The figure shows three views and two pictorial views of one solid part (mm, origin at its lowest corner). Answer the questions. Coordinates: 2 decimals unless noted, no trailing zeros. Order: outer loops, then holes, each group sorted by start corner. A loop starts at its lowest first (then second) coordinate and runs counter-clockwise, first axis right, second up. Notation, with made-up numbers: (80, 76.5) -> (111, 76.5) arc R32 ccw to (111, 105.5) -> close; hole circle Ø2 at (62.5, 20). An arc over 180 degrees is marked (long way). Use one line per item in the form item = value.
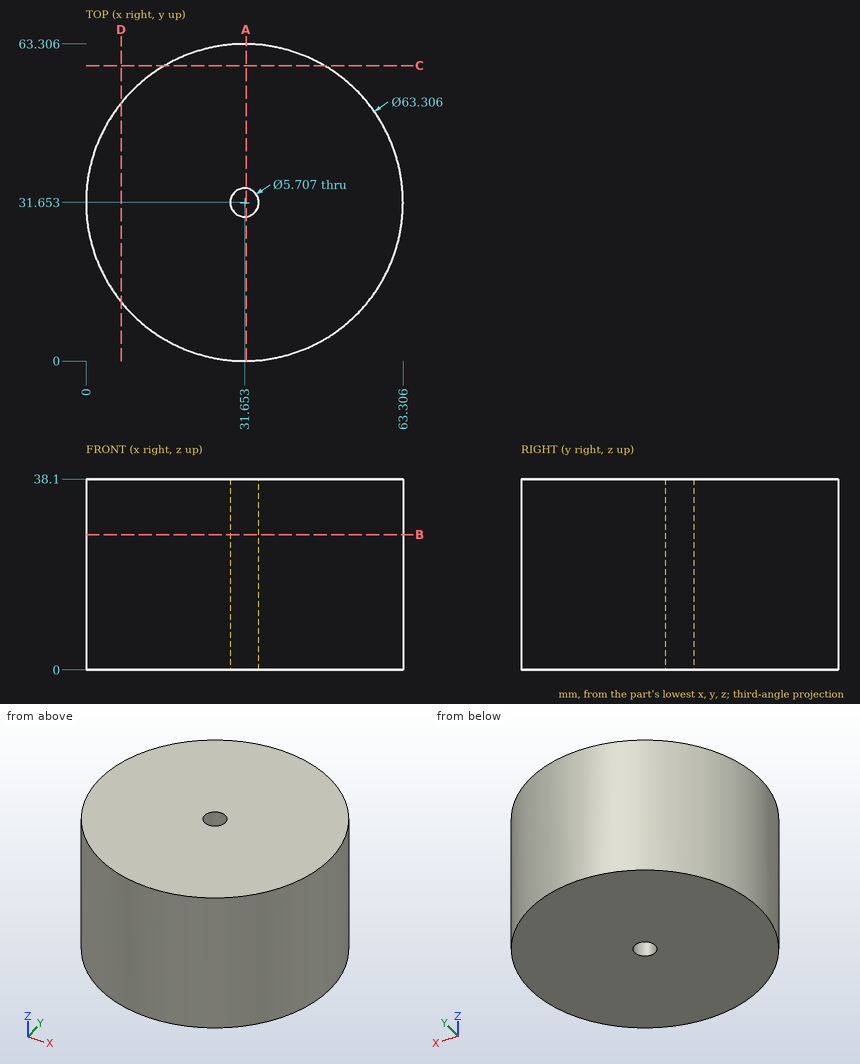
(1) Straight lines are drawn through the part: line 1 along X through (y, z) = (30.5, 18) (1 decimal); line 2 along Y through (x, z) = (33, 24); line 3 along X through (y, z) = (30, 7.5). For each, find the intervals that lie inside material, in ascending order.
Data:
line_1 = 0 to 29, 34.3 to 63.3
line_2 = 0.03 to 29.14, 34.17 to 63.28
line_3 = 0.04 to 29.33, 33.98 to 63.26
(2) Section A-A on x = 32 is taken. Write down the section's boundary in (y, z).
Data:
outline = (0, 0) -> (28.82, 0) -> (28.82, 38.1) -> (0, 38.1) -> close; (34.49, 0) -> (63.3, 0) -> (63.3, 38.1) -> (34.49, 38.1) -> close
(3) Section C-C on y = 59 is taken. Write down the section's boundary in (x, z), plus the area to 3 significant figures.
Data:
outline = (15.71, 0) -> (47.59, 0) -> (47.59, 38.1) -> (15.71, 38.1) -> close
area = 1,210 mm²
(4) Each of these flat-tipped pins is pushed along its axis until it touches: P1, Ø6, axis at y = 23.5, z = 4.5, coming from the +X side; P2, Ø1, axis at y = 9.5, z = 7.5, coming from the +X side; P3, Ø5, axis at y = 22, z = 17.5, coming from the -X side; P4, Ø5, axis at x = 36, y = 32, coming from the -Z side. Where does it stop, or does it pass through?
Data:
P1 = 62.88
P2 = 54.74
P3 = 0.82
P4 = 0
(5) Section B-B on z = 27 is taken. Write down the section's boundary in (x, y).
Data:
outline = circle Ø63.31 at (31.65, 31.65); hole circle Ø5.71 at (31.65, 31.65)
(6) Section D-D on x = 7 is taken. Write down the section's boundary in (y, z), plus the area to 3 significant figures.
Data:
outline = (11.8, 0) -> (51.51, 0) -> (51.51, 38.1) -> (11.8, 38.1) -> close
area = 1,510 mm²
